Can you work these out from the model? Positions are in its coordinate system, mm. A direction names the side the tool comes from. Give positions to 0.01 mm unless a question says otherwise; leave off trailing zeros. Loops run counter-clockwise (first coordinate to the right, second up) from the corner with the lowest first, then second, coordinate; pieces in that order, holes last. Notation, with made-up numbers: M 77.5,39 L 134.5,39 A13 cw 134.5,63 Z; hole C 20.25,14.25 d5. An arc over 180 degrees is marked long. Answer as a JSON object with one key per item and string values.
```python
from build123d import *

# Parameters (mm, degrees)
SKETCH1_R           = 6.5
SKETCH1_R_2         = 2.5
BOSS_EXTRUDE1_DEPTH = 18
SKETCH2_R           = 6.5
SKETCH2_R_2         = 4.9
CUT_EXTRUDE1_DEPTH  = 11


with BuildPart() as part:
    # Sketch1 → Boss-Extrude1 (new body)
    with BuildSketch(Plane(origin=(0, 0, 0), x_dir=(0, 0, -1), z_dir=(1, 0, 0))):
        Circle(SKETCH1_R)
        Circle(SKETCH1_R_2, mode=Mode.SUBTRACT)
    extrude(amount=BOSS_EXTRUDE1_DEPTH)

    # Sketch2 → Cut-Extrude1 (cut)
    with BuildSketch(Plane.ZY.offset(-1)):
        Circle(SKETCH2_R)
        Circle(SKETCH2_R_2, mode=Mode.SUBTRACT)
    extrude(amount=-CUT_EXTRUDE1_DEPTH, mode=Mode.SUBTRACT)


solid = part.part
```
1) For faces 1 (the cylindrical face through (6.423, -4.783, -1.062)), 2 (the flat face through (18, 0, -3)), which set-ups out of +Z, -Z, +X, -X, +Y, -Y let a thin tool reach every point of the face, with its end or its side?
Answer list:
{"face 1": "none", "face 2": "+Z, -Z, +X, +Y, -Y"}
2) Suppose I cut it at A-A, the plane z = 0. Write out the boundary of the cut face in (x, y).
Answer list:
{"outline": "M 0,-6.5 L 1,-6.5 L 1,-4.9 L 12,-4.9 L 12,-6.5 L 18,-6.5 L 18,-2.5 L 0,-2.5 Z; M 0,2.5 L 18,2.5 L 18,6.5 L 12,6.5 L 12,4.9 L 1,4.9 L 1,6.5 L 0,6.5 Z"}
3) Suppose I cut it at D-D, the plane z = 4.5. Write out the boundary of the cut face in (x, y).
Answer list:
{"outline": "M 0,-4.69 L 1,-4.69 L 1,-1.94 L 12,-1.94 L 12,-4.69 L 18,-4.69 L 18,4.69 L 12,4.69 L 12,1.94 L 1,1.94 L 1,4.69 L 0,4.69 Z"}
4) Suppose I cut it at C-C, the plane x = 9.75. Write out the boundary of the cut face in (y, z).
Answer list:
{"outline": "C 0,0 d9.8; hole C 0,0 d5"}
5) Please list where these lines run through material, in increasing order: line 1 along X through (y, z) = (-2.75, -5); line 2 along Y through (x, z) = (12.25, 0); line 3 along Y through (x, z) = (6, 0). Write a range as from..to.
Answer list:
{"line 1": "0..1, 12..18", "line 2": "-6.5..-2.5, 2.5..6.5", "line 3": "-4.9..-2.5, 2.5..4.9"}
6) Will these pins go through, and if not, where does the flat tip stop? pin 1 Ø1.5 at (x, z) = (7, -2) entering from -Y; pin 2 Ø1.5 at (x, z) = (4, 1.5) entering from +Y; pin 3 Ø4 at (x, y) = (9.5, 2) entering from +Z; pin 4 Ø6.5 at (y, z) = (-0.5, 0) entering from +X.
Answer list:
{"pin 1": "y = -4.74", "pin 2": "y = 4.84", "pin 3": "z = 4.9", "pin 4": "x = 18"}
7) Suppose I cut it at B-B, the plane y = -1.75. Write out the boundary of the cut face in (x, z).
Answer list:
{"outline": "M 0,-6.26 L 1,-6.26 L 1,-4.58 L 12,-4.58 L 12,-6.26 L 18,-6.26 L 18,-1.79 L 0,-1.79 Z; M 0,1.79 L 18,1.79 L 18,6.26 L 12,6.26 L 12,4.58 L 1,4.58 L 1,6.26 L 0,6.26 Z"}
8) If we mould it in two halves opening along X, with no side actions, what happens to faces 3 (the cylindrical face through (0.493, -3.955, 5.158)), 4 (the flat face through (12, 5, 1)), 5 (the flat face through (0, 0, -3)), 6 (the flat face through (1, 5, 1))? For each: +X half, -X half, draft (parallel to the pull), parting line (faces both ways), or undercut.
Answer list:
{"face 3": "draft", "face 4": "undercut", "face 5": "-X half", "face 6": "undercut"}
